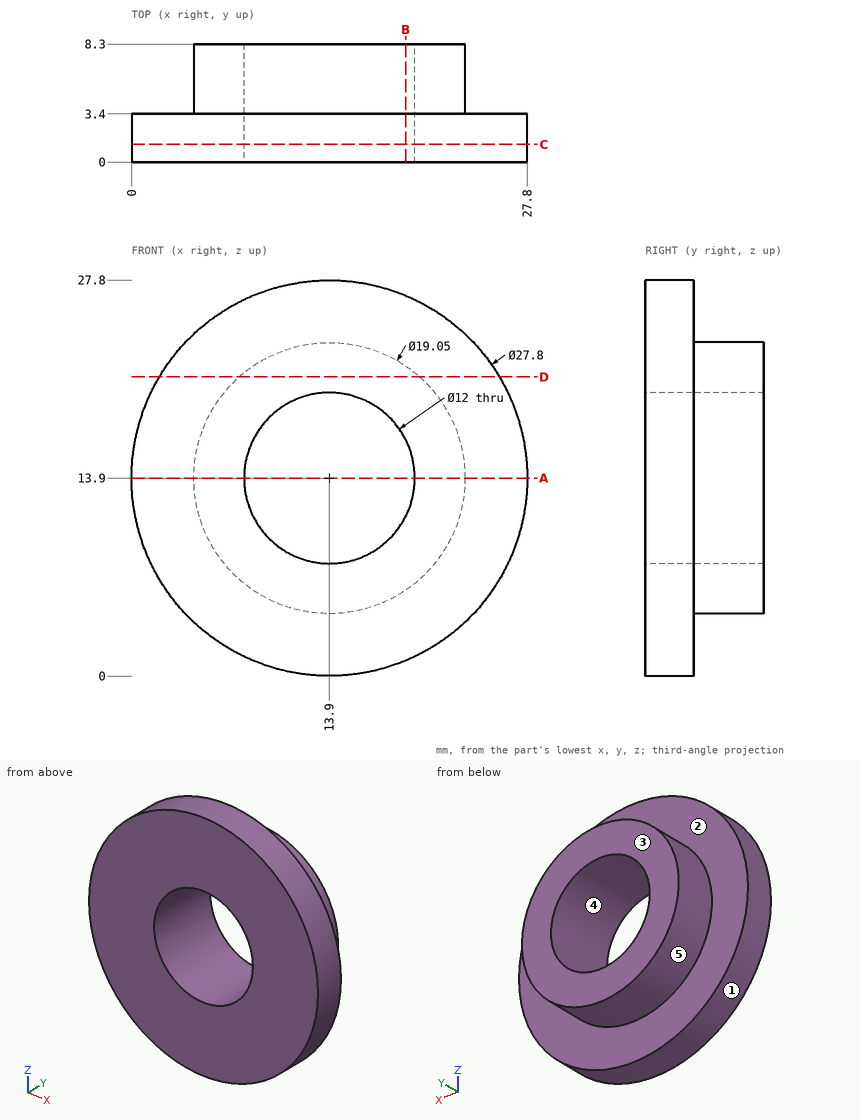
Could you check a few things on this drawing? It's one solid part, dimensions in mm from its lowest x, y, z. A direction names the side the tool comes from. Give positions to 0.01 mm unless a question says otherwise; leave off trailing zeros. Order: outer loops, then holes, each group sorted by start corner. A loop starts at its lowest first (then second) coordinate and runs counter-clockwise, first axis right, second up. Notation, with made-up numbers: (75.25, -29.5) -> (118.25, -29.5) arc R35 cw to (118.25, 7.5) -> close; hole circle Ø2 at (35, 40). An arc over 180 degrees is marked (long way). Answer in a Markdown table with one row per item. Add a question column.
Item 1: Imagine slicing it at B-B (x = 19.25). List the corners of the cut face in (y, z) for me, and give its area (3 significant figures).
Item 2: I'm going to push flat-ended pins straight in: P1, Ø4, axis at x = 20.5, y = 6.5, coming from the +Z side; P2, Ø2, axis at x = 5, y = 1, coming from the -Z side; P3, Ø1, axis at y = 5, z = 22.5, coming from the -X side. Where does each tip first touch, or does it pass through?
Item 3: Imagine slicing it at A-A (z = 13.9). List the corners of the cut face in (x, y) for me (3 decimals).
Item 4: For the marked faces 1 and 2, which set-ups out of +Z, -Z, +X, -X, +Y, -Y let a thin tool reach every point of the face, with its end or its side?
Item 5: Imagine slicing it at D-D (z = 21). List the corners of the cut face in (x, y) for me.
Item 6: Please list where these lines run through material, in increasing order: probe 1 along Z at (x, y) = (13.75, 7); probe 2 along X at (y, z) = (0.5, 8.5); probe 3 along Y at (x, z) = (26.5, 15).
Item 7: We'd pull the mould along Z, two halves only. Please class the marked faces 3, 4 and 5: pulls with the +Z half, pulls with the -Z half, needs draft (parallel to the pull), parting line crosses it, or undercut.
Item 8: Imagine slicing it at C-C (y = 1.25). List the corners of the cut face in (x, z) for me, and give its area (3 significant figures).
Result:
| question | item | result |
|---|---|---|
| 1 | outline | (0, 1.07) -> (3.4, 1.07) -> (3.4, 6.02) -> (8.3, 6.02) -> (8.3, 11.18) -> (0, 11.18) -> close; (0, 16.62) -> (8.3, 16.62) -> (8.3, 21.78) -> (3.4, 21.78) -> (3.4, 26.73) -> (0, 26.73) -> close |
| 1 | area | 119 mm2 |
| 2 | P1 | z = 22.24 |
| 2 | P2 | z = 2.46 |
| 2 | P3 | x = 8.89 |
| 3 | outline | (0, 0) -> (7.9, 0) -> (7.9, 8.3) -> (4.375, 8.3) -> (4.375, 3.4) -> (0, 3.4) -> close; (19.9, 0) -> (27.8, 0) -> (27.8, 3.4) -> (23.425, 3.4) -> (23.425, 8.3) -> (19.9, 8.3) -> close |
| 4 | face 1 | +Y, -Y |
| 4 | face 2 | +Y |
| 5 | outline | (1.95, 0) -> (25.85, 0) -> (25.85, 3.4) -> (20.25, 3.4) -> (20.25, 8.3) -> (7.55, 8.3) -> (7.55, 3.4) -> (1.95, 3.4) -> close |
| 6 | probe 1 | 4.38 to 7.9, 19.9 to 23.42 |
| 6 | probe 2 | 1.09 to 11.28, 16.52 to 26.71 |
| 6 | probe 3 | 0 to 3.4 |
| 7 | face 3 | needs draft |
| 7 | face 4 | undercut |
| 7 | face 5 | parting line crosses it |
| 8 | outline | circle Ø27.8 at (13.9, 13.9); hole circle Ø12 at (13.9, 13.9) |
| 8 | area | 494 mm2 |
